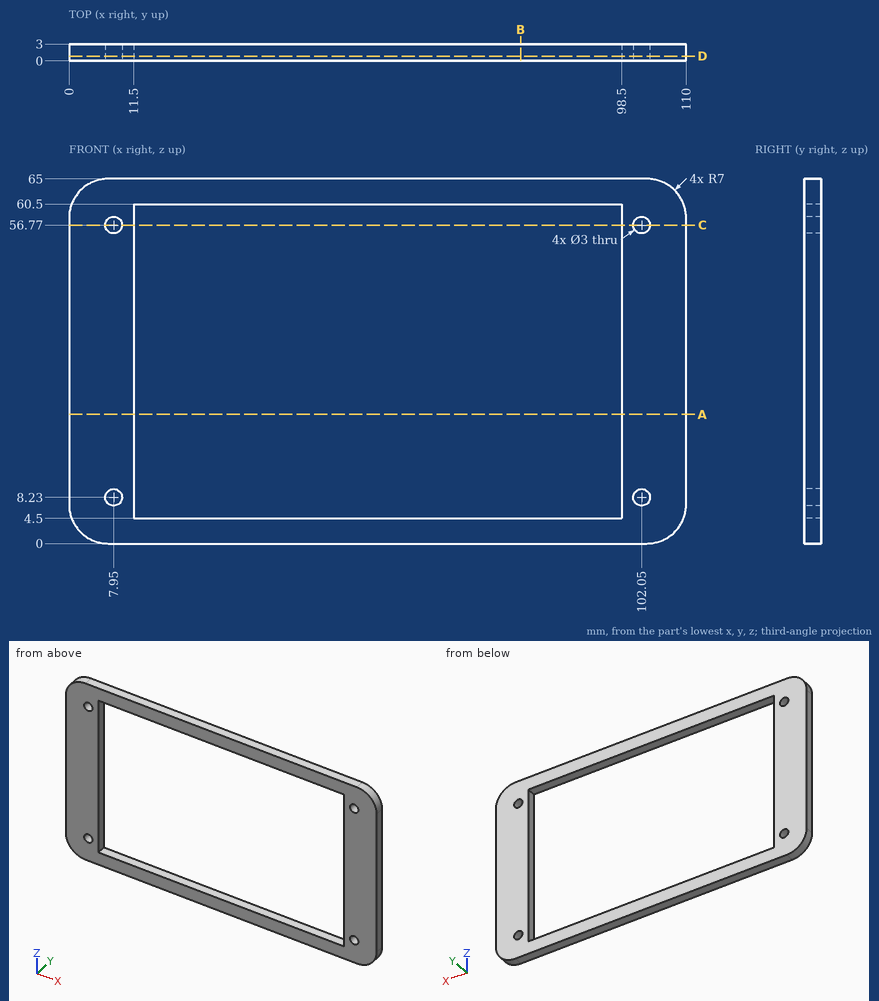
Here's the drawing with two shaded views (mm, measured from the low corner). I have some questions. Give positions to 0.01 mm unless a question says otherwise; leave off trailing zeros. Order: outer loops, then holes, each group sorted by start corner. A loop starts at its lowest first (then second) coordinate and runs counter-clockwise, first axis right, second up. Notation, with made-up numbers: (12.5, -24.75) - (52.5, -24.75) arc R7 cw to (52.5, -15.75) - close; hole circle Ø2 at (47, 69.25). An arc over 180 degrees is marked (long way). Use a Markdown table: item, result. Add a question column.
Q1. Please list where these lines run through material, in increasing order: line 1 along X through (y, z) = (1.15, 56.77); line 2 along Z through (x, y) = (33, 2.6); line 3 along X through (y, z) = (0.95, 32.5).
Q2. If we section it at C-C on z = 56.77: Write out the boundary of the cut face in (x, y), plus the area to 3 significant figures.
Q3. I'm going to push a flat-ended pin straight in: pin 1 (2.5 mm diameter, centred on x = 102.05, z = 56.77, fed in from +Y). Where does the tip first touch, or does it pass through?
Q4. If we section it at D-D on y = 0.85: Write out the boundary of the cut face in (x, z).
Q5. If we section it at B-B on x = 80.5: Write out the boundary of the cut face in (y, z), plus the area to 3 significant figures.
Q6. If we section it at A-A on z = 23: Write out the boundary of the cut face in (x, y), plus the area to 3 significant figures.
Answers follow:
| question | item | result |
|---|---|---|
| 1 | line 1 | x = 0 to 6.45, 9.45 to 11.5, 98.5 to 100.55, 103.55 to 110 |
| 1 | line 2 | z = 0 to 4.5, 60.5 to 65 |
| 1 | line 3 | x = 0 to 11.5, 98.5 to 110 |
| 2 | outline | (0, 0) - (6.45, 0) - (6.45, 3) - (0, 3) - close; (9.45, 0) - (11.5, 0) - (11.5, 3) - (9.45, 3) - close; (98.5, 0) - (100.55, 0) - (100.55, 3) - (98.5, 3) - close; (103.55, 0) - (110, 0) - (110, 3) - (103.55, 3) - close |
| 2 | area | 51.0 mm^2 |
| 3 | pin 1 | passes through |
| 4 | outline | (0, 7) arc R7 ccw to (7, 0) - (103, 0) arc R7 ccw to (110, 7) - (110, 58) arc R7 ccw to (103, 65) - (7, 65) arc R7 ccw to (0, 58) - close; hole circle Ø3 at (7.95, 8.23); hole circle Ø3 at (7.95, 56.77); hole (11.5, 4.5) - (98.5, 4.5) - (98.5, 60.5) - (11.5, 60.5) - close; hole circle Ø3 at (102.05, 8.23); hole circle Ø3 at (102.05, 56.77) |
| 5 | outline | (0, 0) - (3, 0) - (3, 4.5) - (0, 4.5) - close; (0, 60.5) - (3, 60.5) - (3, 65) - (0, 65) - close |
| 5 | area | 27.0 mm^2 |
| 6 | outline | (0, 0) - (11.5, 0) - (11.5, 3) - (0, 3) - close; (98.5, 0) - (110, 0) - (110, 3) - (98.5, 3) - close |
| 6 | area | 69.0 mm^2 |
